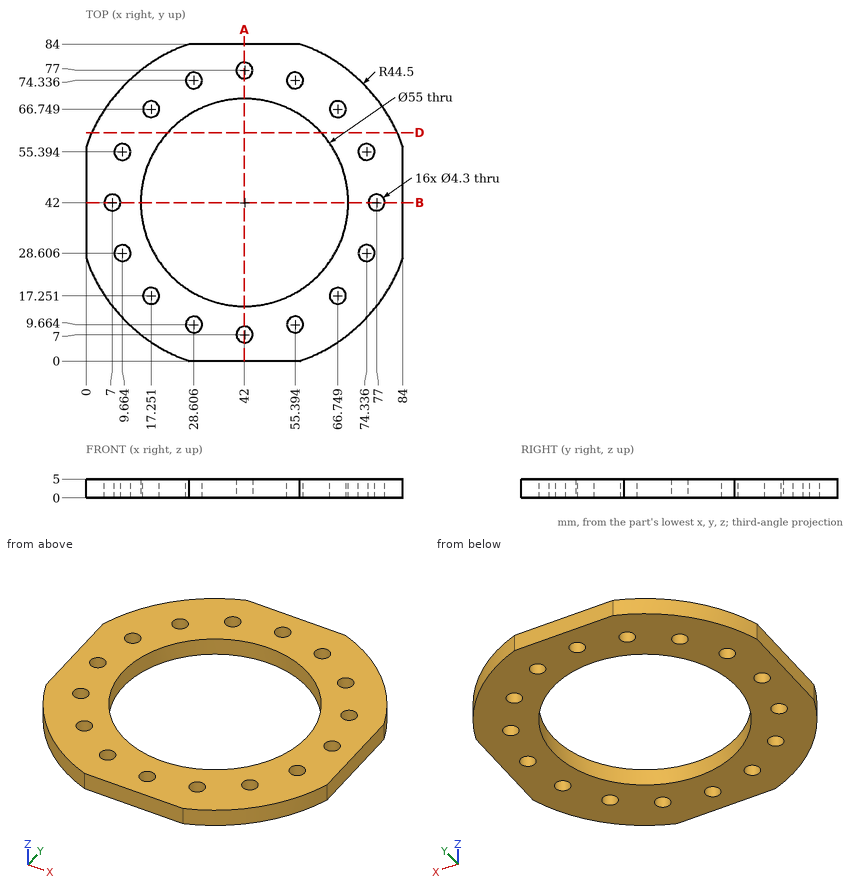
The figure shows three views and two pictorial views of one solid part (mm, origin at its lowest corner). Answer the questions. Give positions to 0.01 mm unless a question says otherwise; leave off trailing zeros. Write each loop counter-clockwise with the first axis right and the second up, starting at its lowest first coordinate (ties: lowest second). Pieces come first, ordered by that corner, then holes. Notation, with made-up numbers: (40.5, 79.25) - (98.5, 79.25) arc R19 ccw to (98.5, 97.25) - close; hole circle Ø9 at (67, 6). An arc over 180 degrees is marked (long way). Use one line per item in the form item = value. Start each with the question number.
1) Find section D-D on y = 60.5. Determine the outline of the cut face in (x, z), plus the area to 3 significant figures.
2) Flat-ended cylindrical pins translate along their axes: pin 1 Ø3.5 at (x, y) = (42, 7) entering from +Z; pin 2 Ø3 at (y, z) = (60.5, 3.5) entering from -X (1 decimal). Find the tip coordinate at first contact, or state that the pin passes through.
3) Consider line 1 along Y through (x, z) = (42, 0.8); line 2 along X through (y, z) = (43.5, 3.7); line 3 along Y through (x, z) = (55, 1.65). Determine where each line is inside the solid, lowest interval first. Write a range as from..to.
4) Find section A-A on x = 42. Determine the outline of the cut face in (y, z), plus the area to 3 significant figures.
Geometry results:
q1.outline = (1.53, 0) - (21.65, 0) - (21.65, 5) - (1.53, 5) - close; (62.35, 0) - (82.47, 0) - (82.47, 5) - (62.35, 5) - close
q1.area = 201 mm2
q2.pin_1 = through
q2.pin_2 = 0.9
q3.line_1 = 0..4.85, 9.15..14.5, 69.5..74.85, 79.15..84
q3.line_2 = 0..5.46, 8.54..14.54, 69.46..75.46, 78.54..84
q3.line_3 = 0..7.55, 11.78..17.77, 66.23..72.22, 76.45..84
q4.outline = (0, 0) - (4.85, 0) - (4.85, 5) - (0, 5) - close; (9.15, 0) - (14.5, 0) - (14.5, 5) - (9.15, 5) - close; (69.5, 0) - (74.85, 0) - (74.85, 5) - (69.5, 5) - close; (79.15, 0) - (84, 0) - (84, 5) - (79.15, 5) - close
q4.area = 102 mm2
